Model file for the job. Use its own axes, mm. Face numbers are marked on the shaded views. A direction names the side the tool comes from. Coordinates: 2 decimals unless noted, no trailing zeros. Order: outer loops, then holes, each group sorted by start corner. A loop starts at its lowest first (then second) coordinate and runs counter-clockwise, first axis right, second up.
from build123d import *

# Parameters (mm, degrees)
SKETCH2_W           = 50
SKETCH2_H           = 35
BOSS_EXTRUDE1_DEPTH = 50
SKETCH3_W           = 40.72
SKETCH3_H           = 20.17
CUT_EXTRUDE1_DEPTH  = 28.82
BOSS_EXTRUDE2_DEPTH = 35
SKETCH5_R           = 4.817251836
CUT_EXTRUDE2_DEPTH  = 5.82


with BuildPart() as part:
    # Sketch2 → Boss-Extrude1 (new body)
    with BuildSketch(Plane.XY):
        Rectangle(SKETCH2_W, SKETCH2_H)
    extrude(amount=BOSS_EXTRUDE1_DEPTH)

    # Sketch3 → Cut-Extrude1 (cut)
    with BuildSketch(Plane.XY.offset(50)):
        Rectangle(SKETCH3_W, SKETCH3_H)
    extrude(amount=-CUT_EXTRUDE1_DEPTH, mode=Mode.SUBTRACT)

    # Sketch4 → Boss-Extrude2 (add)
    with BuildSketch(Plane(origin=(0, 17.5, 0), x_dir=(1, 0, 0), z_dir=(0, 1, 0))):
        Polygon((25, -50), (25, 0), (25, 10), (85, 10), (85, 0), (35, 0), (35, -50), (85, -50), (85, -60), (25, -60), align=None)
    extrude(amount=-BOSS_EXTRUDE2_DEPTH)

    # Sketch5 → Cut-Extrude2 (cut)
    with BuildSketch(Plane.XY):
        with Locations((67.294168967, 0)):
            Circle(SKETCH5_R)
    extrude(amount=-CUT_EXTRUDE2_DEPTH, mode=Mode.SUBTRACT)


solid = part.part
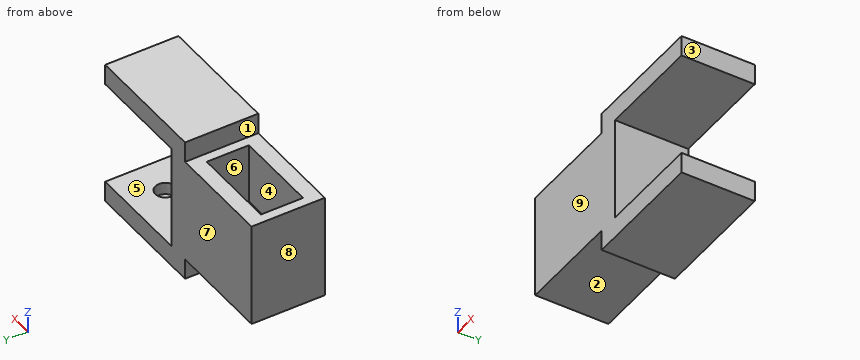
Q1. Mould opens along Y. For the marked faces 6, 7, 8 and 9 say: pulls with the +Y half, pulls with the -Y half, needs draft (parallel to the pull), parting line crosses it, or undercut.
Established:
face 6: undercut
face 7: pulls with the +Y half
face 8: needs draft
face 9: pulls with the -Y half
Q2. Cut at C-C, the plane y = -13. List the corners of the cut face in (x, z).
Established:
outline: (-25, 0) - (25, 0) - (25, -10) - (85, -10) - (85, 0) - (35, 0) - (35, 50) - (85, 50) - (85, 60) - (25, 60) - (25, 50) - (-25, 50) - close
Q3. Which spindle directions (+Z, -Z, +X, -X, +Y, -Y) get a long thin tool onto all of the face, cutting with end or side? Do the marked faces 1, 2, 3, 4 and 5. Say none if no direction does.
Established:
face 1: +Z, -X, +Y, -Y
face 2: -Z, -X, +Y, -Y
face 3: +Z, -Z, +X, +Y, -Y
face 4: +Z
face 5: +X, +Y, -Y
Q4. Cut at B-B, the plane z = 42. List the corners of the cut face in (x, y) (3 decimals).
Established:
outline: (-25, -17.5) - (35, -17.5) - (35, 17.5) - (-25, 17.5) - close; hole (-20.36, -10.085) - (20.36, -10.085) - (20.36, 10.085) - (-20.36, 10.085) - close
Q5. Drop flat-ended pins along their axis: P1, Ø6, axis at y = -3, z = 31, coming from the +X side; P2, Ø17.5, axis at x = 3.5, y = -7, coming from the +Z side; P3, Ø6, axis at x = 10, y = -4, coming from the +Z side. Give the stop position or say it passes through.
Established:
P1: stops at x = 35
P2: stops at z = 50
P3: stops at z = 21.18
Q6. Probe line 1 (X direction, y = 7, z = 39); line 2 (Z direction, x = 36, y = -8.5); line 3 (Y direction, x = 17.5, z = 30.5) (3 decimals). List the from-to ranges inside material, lowest first.
Established:
line 1: x = -25 to -20.36, 20.36 to 35
line 2: z = -10 to 0, 50 to 60
line 3: y = -17.5 to -10.085, 10.085 to 17.5
Q7. Cut at A-A, the plane x = 78.5. List the corners of the cut face in (y, z).
Established:
outline: (-17.5, -10) - (17.5, -10) - (17.5, 0) - (-17.5, 0) - close; (-17.5, 50) - (17.5, 50) - (17.5, 60) - (-17.5, 60) - close
